from build123d import *

# Parameters (mm, degrees)
F0_R     = 3.175
F1_DEPTH = 3.048


with BuildPart() as f1:
    # F0 (on Front) → F1 (new body)
    with BuildSketch(Plane.XZ):
        with BuildLine():
            ThreePointArc((0.67949, -9.500732), (6.97129, -6.490511), (9.525, 0))
            ThreePointArc((9.525, 0), (0, 9.525), (-9.525, 0))
            ThreePointArc((-9.525, 0), (-6.735192, -6.735192), (0, -9.525))
            Line((0, -9.525), (0.67949, -9.500732))
        make_face()
        Circle(F0_R, mode=Mode.SUBTRACT)
        with BuildLine():
            ThreePointArc((-9.525, 0), (0, 9.525), (9.525, 0))
            ThreePointArc((9.525, 0), (6.97129, -6.490511), (0.67949, -9.500732))
            Line((0.67949, -9.500732), (44.45, -7.9375))
            ThreePointArc((44.45, -7.9375), (36.5125, 0), (44.45, 7.9375))
            Line((44.45, 7.9375), (17.946122, 7.9375))
            ThreePointArc((17.946122, 7.9375), (11.979481, 10.633666), (10.059795, 16.893451))
            Line((10.059795, 16.893451), (15.747457, 61.491711))
            ThreePointArc((15.747457, 61.491711), (0, 47.625), (-15.747457, 61.491711))
            Line((-15.747457, 61.491711), (-9.525, 0))
        make_face()
        with BuildLine():
            ThreePointArc((0, -9.525), (0.339962, -9.518931), (0.67949, -9.500732))
            Line((0.67949, -9.500732), (0, -9.525))
        make_face()
        with BuildLine():
            ThreePointArc((-15.747457, 65.508289), (-15.875, 63.5), (-15.747457, 61.491711))
            ThreePointArc((-15.747457, 61.491711), (0, 47.625), (15.747457, 61.491711))
            ThreePointArc((15.747457, 61.491711), (15.843082, 62.493832), (15.875, 63.5))
            ThreePointArc((15.875, 63.5), (15.843082, 64.506168), (15.747457, 65.508289))
            ThreePointArc((15.747457, 65.508289), (0, 79.375), (-15.747457, 65.508289))
        make_face()
        with Locations((0, 63.5)):
            Circle(F0_R, mode=Mode.SUBTRACT)
        with BuildLine():
            ThreePointArc((44.45, 7.9375), (36.5125, 0), (44.45, -7.9375))
            ThreePointArc((44.45, -7.9375), (50.06266, -5.61266), (52.3875, 0))
            ThreePointArc((52.3875, 0), (50.06266, 5.61266), (44.45, 7.9375))
        make_face()
        with Locations((44.45, 0)):
            Circle(F0_R, mode=Mode.SUBTRACT)
        with BuildLine():
            Line((-9.525, 114.3), (-15.747457, 65.508289))
            ThreePointArc((-15.747457, 65.508289), (0, 79.375), (15.747457, 65.508289))
            Line((15.747457, 65.508289), (9.525, 114.3))
            ThreePointArc((9.525, 114.3), (0, 104.775), (-9.525, 114.3))
        make_face()
        with Locations((-1.5875, 100.0252)):
            Circle(F0_R, mode=Mode.SUBTRACT)
        with BuildLine():
            ThreePointArc((9.525, 114.3), (0, 123.825), (-9.525, 114.3))
            ThreePointArc((-9.525, 114.3), (0, 104.775), (9.525, 114.3))
        make_face()
        with Locations((0, 114.3)):
            Circle(F0_R, mode=Mode.SUBTRACT)
    extrude(amount=-F1_DEPTH)


solid = f1.part
Geometry: final body of the model. Coordinates: model frame, mm. A direction names the side the tool comes from. Give positions to 0.01 mm unless a question says otherwise; leave off trailing zeros. Loops run counter-clockwise (first coordinate to the right, second up) from the corner with the lowest first, then second, coordinate; pieces in that order, holes last. Notation, with made-up numbers: M 63.5,17.5 L 84.5,17.5 A6 cw 84.5,22.5 Z; hole C -17.5,-6 d1. An arc over 180 degrees is marked long. Put each result on its own line as item: value.
1) Mould query, pull axis Z, two halves, no side actions, for faces 4 (the cylindrical face through (0.209, 1.503, 123.823)), 5 (the cylindrical face through (-15.875, 1.503, 63.528)), 6 (the cylindrical face through (12.042, 1.503, 10.563)). Classes: released by +Z, released by -Z, zero draft, split by the parting line, or undercut.
Computed values:
face 4: released by +Z
face 5: split by the parting line
face 6: undercut
2) Cut plane B-B, the plane z = 48. Return the cut outline in (x, y).
Computed values:
outline: M -14.38,0 L 14.03,0 L 14.03,3.05 L -14.38,3.05 Z
3) Cut plane C-C, the plane x = 19.5. Return the cut outline in (y, z), plus the area to 3 significant figures.
Computed values:
outline: M 0,-8.83 L 3.05,-8.83 L 3.05,7.94 L 0,7.94 Z
area: 51.1 mm^2
4) Cut plane A-A, the plane y = 2.5. Give the number of separate pieces and of enclosed holes in the cut face, plus the area to 3 significant figures.
Computed values:
separate pieces: 1
enclosed holes: 5
area: 3,710 mm^2
5) Reachability of faces 1 (the flat face through (31, 2, 7.938)), 2 (the cylindrical face through (1.707, 1.503, 66.177)), 3 (the flat face through (12.864, 1.503, 38.88)) from +Z, -Z, +X, -X, +Y, -Y: full face, straight path, thin tool, end or side. Return the list, or none.
Computed values:
face 1: +Z, +X, +Y, -Y
face 2: +Y, -Y
face 3: +X, +Y, -Y
6) Material intervals for L1, parallel to Z at x = 44, y = 0.3; L2, parallel to X at y = 0.65, z = 58; L3, parallel to X at y = 2.25, z = 93.5, sorted ascending. Write a range as from..to.
Computed values:
L1: z = -7.95..-3.14, 3.14..7.94
L2: x = -15.39..15.3
L3: x = -12.18..12.18
